Build history of the part. All positions in model axes, mm. Give positions to 0.01 mm unless a question says otherwise; leave off trailing zeros. One line per item, written item: value. Start each with the question number.
(1) Saw through at A-A on z = 2.2. Count the separate pieces of the cut face and the enclosed holes in it, plus the area to 3 significant figures.
(2) Pin check, flat tip, straight feed: pin 1 (3 mm diameter, centred on x = 131.21, y = 20.78, fed in from -Z). Stop position of the tip, or through.
(3) Probe line 1 (Y direction, x = 0.5, z = 2.95); line 2 (X direction, y = -1.5, z = 0.45); line 3 (Y direction, x = 20.5, z = 1.15). List the from-to ranges inside material, lowest first.
```python
from build123d import *

# Parameters (mm, degrees)
SKETCH1_R           = 187.5
BOSS_EXTRUDE1_DEPTH = 4
SKETCH2_R           = 37.5
CUT_EXTRUDE1_DEPTH  = 266.195211118
SKETCH3_R           = 1.755
CUT_EXTRUDE2_DEPTH  = 266.195211118
CIRPATTERN1_COUNT   = 20
SKETCH4_R           = 1.755
CUT_EXTRUDE3_DEPTH  = 266.195211118
CIRPATTERN2_COUNT   = 20


with BuildPart() as part:
    # Sketch1 → Boss-Extrude1 (new body)
    with BuildSketch(Plane.XY):
        Circle(SKETCH1_R)
    extrude(amount=BOSS_EXTRUDE1_DEPTH)

    # Sketch2 → Cut-Extrude1 (cut, through all)
    with BuildSketch(Plane.XY.offset(4)):
        Circle(SKETCH2_R)
    extrude(amount=-CUT_EXTRUDE1_DEPTH, mode=Mode.SUBTRACT)

    # Sketch3 → Cut-Extrude2 (cut, through all)
    with BuildSketch(Plane.XY.offset(4)):
        with Locations((0, 175)):
            Circle(SKETCH3_R)
    cut_extrude2 = extrude(amount=-CUT_EXTRUDE2_DEPTH, mode=Mode.SUBTRACT)

    # CirPattern1: Cut-Extrude2 ×20 about axis
    cirpattern1_axis = Axis((0, 0, 0), (0, 0, 1))
    for i in range(1, CIRPATTERN1_COUNT):
        add(cut_extrude2.rotate(cirpattern1_axis, i * 360 / CIRPATTERN1_COUNT), mode=Mode.SUBTRACT)

    # Sketch4 → Cut-Extrude3 (cut, through all)
    with BuildSketch(Plane.XY.offset(4)):
        with Locations((73.815845007, 37.611051607)):
            Circle(SKETCH4_R)
        with Locations((118.366171216, 60.310576594)):
            Circle(SKETCH4_R)
    cut_extrude3 = extrude(amount=-CUT_EXTRUDE3_DEPTH, mode=Mode.SUBTRACT)

    # CirPattern2: Cut-Extrude3 ×20 about axis
    cirpattern2_axis = Axis((0, 0, 0), (0, 0, 1))
    for i in range(1, CIRPATTERN2_COUNT):
        add(cut_extrude3.rotate(cirpattern2_axis, i * 360 / CIRPATTERN2_COUNT), mode=Mode.SUBTRACT)


solid = part.part
```
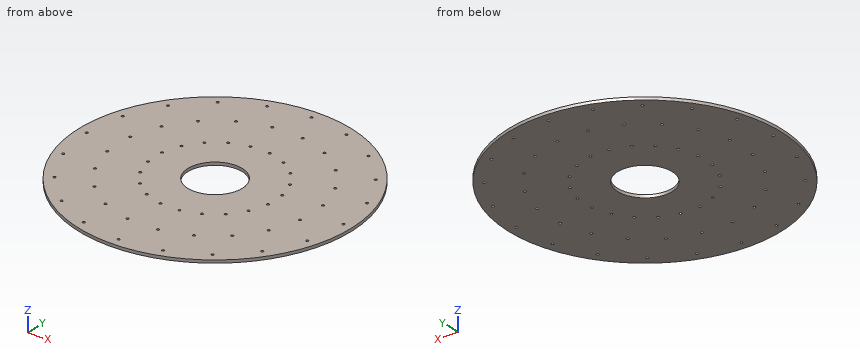
Results below:
1. separate pieces: 1
1. enclosed holes: 61
1. area: 105,000 mm²
2. pin 1: passes through
3. line 1: y = -187.5 to -176.68, -173.32 to -37.5, 37.5 to 173.32, 176.68 to 187.5
3. line 2: x = -187.49 to -175.91, -174.09 to -37.47, 37.47 to 174.09, 175.91 to 187.49
3. line 3: y = -186.38 to -132.94, -129.48 to -31.4, 31.4 to 129.48, 132.94 to 186.38
